Input: part model. Units: mm. Frame: model coordinates. A direction names the side the tool comes from. Round coordinates to 2 decimals unless told otherwise and drop trailing zeros. Loops run counter-clockwise (first coordinate to the right, second up) from the corner with the lowest first, then second, coordinate; pieces in that order, holes last. Notation, with made-up numbers: (-22.5, 66) - (7.5, 66) arc R24 ccw to (7.5, 87) - close; hole circle Ø1 at (15.5, -11). An arc over 180 degrees is marked (long way). One line per question, with ' | ' between items. Start each with the question number.
Item 1: Section C-C, the plane y = -8.5. Return loops of the section in (x, z), plus the area to 3 significant figures.
Item 2: Set-up query: faces 1 (the face through (-24, 1, 11)), 2 (the face through (26, 0, 0)), 3 (the face through (0, 2, -4.5)), 4 (the face through (0, 19, 0)). Return all of +Z, -Z, +X, -X, +Y, -Y with unobstructed straight access to the full face (end or side cutting, diameter ignored); none if empty.
Item 3: First-contact query: pin 1 (6.5 mm diameter, centred on x = 3.5, z = 14, fed in from +Y); pin 2 (5 mm diameter, centred on x = -8, y = 18.5, fed in from +Z). Flat tips, straight axial feed; report the tip coordinate or a pass-through.
Item 4: Draft query along Y for faces 5 (the face through (0, 24, 0)), 6 (the face through (0, 25, 1)), 7 (the face through (0, -25, 0)). Return one class per face: pulls with the +Y half, pulls with the -Y half, needs draft (parallel to the pull), parting line crosses it, or undercut.
Item 5: Material intervals for line 1 along X through (y, z) = (-18, -7.5); line 2 along Y through (x, z) = (-3.5, -0.5); line 3 along Z through (x, y) = (-13, 6), sorted ascending.
Item 6: Section B-B, the plane z = -14. Return loops of the section in (x, y), plus the area to 3 significant figures.
Item 7: Section A-A, the plane x = 15. Return loops of the section in (y, z), plus the area to 3 significant figures.
```python
from build123d import *

# Parameters (mm, degrees)
F0_W     = 48
F0_H     = 47
F1_DEPTH = 4.5
F0_H_2   = 3
F2_DEPTH = 17.5


with BuildPart() as f1:
    # F0 (on Top) → F1 (new body, symmetric)
    with BuildSketch(Plane.XY):
        with Locations((0, 1.5)):
            Rectangle(F0_W, F0_H)
        with BuildLine():
            ThreePointArc((-20.5, 19), (-23, 21.5), (-20.5, 24))
            Line((-20.5, 24), (20.5, 24))
            ThreePointArc((20.5, 24), (22.267767, 23.267767), (23, 21.5))
            ThreePointArc((23, 21.5), (22.267767, 19.732233), (20.5, 19))
            Line((20.5, 19), (-20.5, 19))
        make_face(mode=Mode.SUBTRACT)
    extrude(amount=F1_DEPTH, both=True)

    # F0 (on Top) → F2 (join, symmetric)
    with BuildSketch(Plane.XY):
        Polygon((-24, 25), (-26, 25), (-26, -25), (-24, -25), (-24, -22), align=None)
        with Locations((0, -23.5)):
            Rectangle(F0_W, F0_H_2)
        Polygon((26, 25), (24, 25), (24, -22), (24, -25), (26, -25), align=None)
    extrude(amount=F2_DEPTH, both=True)


solid = f1.part
```
Return value:
1) outline: (-26, -17.5) - (-24, -17.5) - (-24, -4.5) - (24, -4.5) - (24, -17.5) - (26, -17.5) - (26, 17.5) - (24, 17.5) - (24, 4.5) - (-24, 4.5) - (-24, 17.5) - (-26, 17.5) - close | area: 572 mm2
2) face 1: +Z, +Y | face 2: +Z, -Z, +X, +Y, -Y | face 3: -Z, +Y | face 4: +Z, -Z
3) pin 1: y = -22 | pin 2: z = 4.5
4) face 5: undercut | face 6: pulls with the +Y half | face 7: pulls with the -Y half
5) line 1: -26 to -24, 24 to 26 | line 2: -25 to 19, 24 to 25 | line 3: -4.5 to 4.5
6) outline: (-26, -25) - (26, -25) - (26, 25) - (24, 25) - (24, -22) - (-24, -22) - (-24, 25) - (-26, 25) - close | area: 344 mm2
7) outline: (-25, -17.5) - (-22, -17.5) - (-22, -4.5) - (19, -4.5) - (19, 4.5) - (-22, 4.5) - (-22, 17.5) - (-25, 17.5) - close; (24, -4.5) - (25, -4.5) - (25, 4.5) - (24, 4.5) - close | area: 483 mm2
